Geometry check sheet. Reference: the model listing, model coordinates, mm. Face numbers are marked on the shaded views. A direction names the side the tool comes from. Round coordinates to 2 decimals unless told otherwise and drop trailing zeros. Write each loop counter-clockwise with the first axis right and the second up, starting at its lowest first coordinate (ties: lowest second). Pieces come first, ordered by that corner, then holes. Notation, with made-up numbers: (-1.5, 78.25) -> (45.5, 78.25) arc R25 ccw to (45.5, 94.25) -> close; hole circle Ø7 at (76, 54). An arc over 180 degrees is marked (long way). Use a Markdown table: item, result.
```python
from build123d import *

# Parameters (mm, degrees)
F1_DEPTH = 20
F2_R     = 8
F3_DEPTH = 4


with BuildPart() as f1:
    # F0 (on Top) → F1 (new body)
    with BuildSketch(Plane.XY):
        with BuildLine():
            Line((-3, 0), (0, 0))
            Line((0, 0), (0, 113.4485357832))
            ThreePointArc((0, 113.4485357832), (1.0855328259, 119.6048983631), (4.2112000239, 125.0187127576))
            Line((4.2112000239, 125.0187127576), (17.9980530712, 141.4492444073))
            Line((17.9980530712, 141.4492444073), (15.6999197419, 143.3776072364))
            Line((15.6999197419, 143.3776072364), (1.9130666945, 126.9470755866))
            ThreePointArc((1.9130666945, 126.9470755866), (-1.7335450365, 120.630958793), (-3, 113.4485357832))
            Line((-3, 113.4485357832), (-3, 0))
        make_face()
    extrude(amount=F1_DEPTH)

    # F2 (on face) → F3 (cut)
    with BuildSketch(Plane(origin=(-61.3865985101, 51.509472169, 0), x_dir=(-0.6427876097, -0.7660444431, 0), z_dir=(-0.7660444431, 0.6427876097, 0))):
        with Locations((-109.9253331743, 10)):
            Circle(F2_R)
    extrude(amount=-F3_DEPTH, mode=Mode.SUBTRACT)


solid = f1.part
```
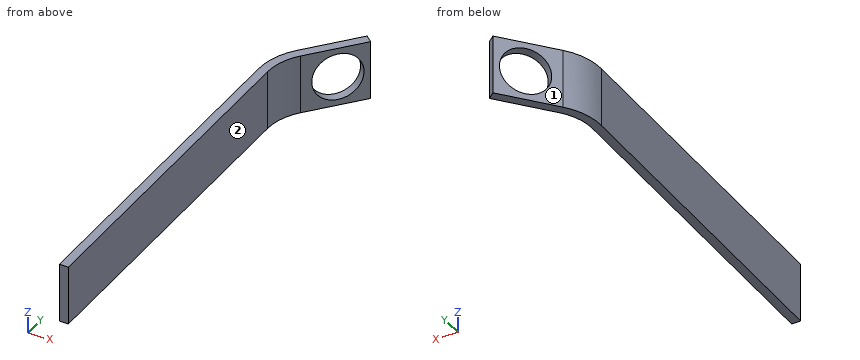
(1) Access from +Z, -Z, +X, -X, +Y, -Y to the whole of each face (thin tool, end or side, straight path). Record for the marked faces 1 and 2.
A:
| item | result |
|---|---|
| face 1 | +Z, -Z, -X, +Y |
| face 2 | +Z, -Z, +X, -Y |
(2) Section check B-B on y = 29. Record the cut outline in (x, z).
A:
| item | result |
|---|---|
| outline | (-3, 0) -> (0, 0) -> (0, 20) -> (-3, 20) -> close |
(3) Gauge pin test, flat ends, axial feed: pin 1 Ø12 at (x, y) = (9.5, 85) entering from -Z; pin 2 Ø6 at (y, z) = (20.5, 10.5) entering from +X. Record the tip position at first contact, or that the pin passes through.
A:
| item | result |
|---|---|
| pin 1 | passes through |
| pin 2 | stops at x = 0 |
(4) Section check C-C on z = 8.5. Record the cut outline in (x, y), plus the area to 3 significant figures.
A:
| item | result |
|---|---|
| outline | (-3, 0) -> (0, 0) -> (0, 113.45) arc R18 cw to (4.21, 125.02) -> (6.52, 127.77) -> (4.22, 129.7) -> (1.91, 126.95) arc R21 ccw to (-3, 113.45) -> close; (14.32, 141.74) -> (16.62, 139.81) -> (18, 141.45) -> (15.7, 143.38) -> close |
| area | 398 mm2 |
(5) Thickness scan on line 1 (X direction, y = 42.5, z = 16); line 2 (Y direction, x = 14.75, z = 5); line 3 (X direction, y = 119.5, z = 18.5). Record the ranges inside material, lowest first.
A:
| item | result |
|---|---|
| line 1 | x = -3 to 0 |
| line 2 | y = 139.27 to 142.25 |
| line 3 | x = -2.11 to 1.05 |
(6) Section check A-A on z = 15.5. Record the cut outline in (x, y), plus the area to 3 significant figures.
A:
| item | result |
|---|---|
| outline | (-3, 0) -> (0, 0) -> (0, 113.45) arc R18 cw to (4.21, 125.02) -> (7.84, 129.34) -> (5.54, 131.27) -> (1.91, 126.95) arc R21 ccw to (-3, 113.45) -> close; (13.01, 140.17) -> (15.3, 138.24) -> (18, 141.45) -> (15.7, 143.38) -> close |
| area | 411 mm2 |
(7) Section check D-D on y = 115.5. Record the cut outline in (x, z), plus the area to 3 significant figures.
A:
| item | result |
|---|---|
| outline | (-2.9, 0) -> (0.12, 0) -> (0.12, 20) -> (-2.9, 20) -> close |
| area | 60.3 mm2 |
